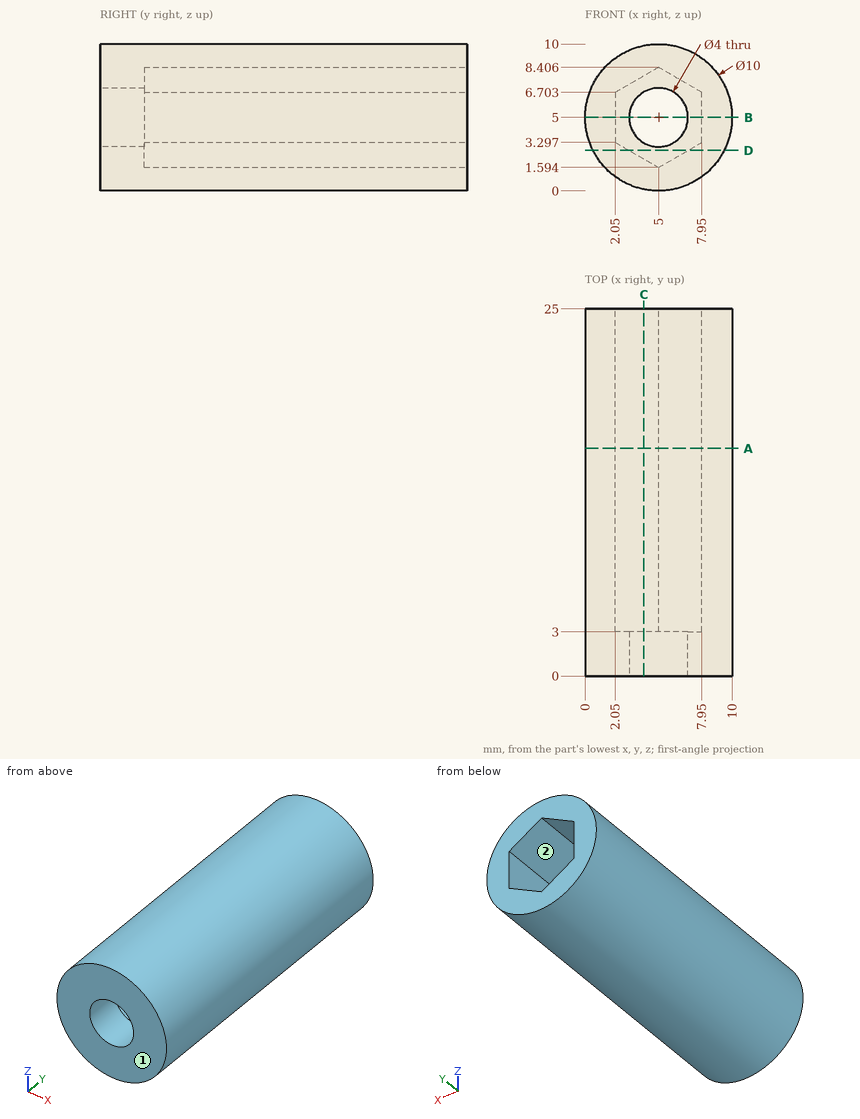
Geometry check sheet. Reference: drawing and pictorial views, mm from the part's lowest x, y, z. A direction names the side the tool comes from. Round coordinates to 2 decimals unless told otherwise and drop trailing zeros. Loops run counter-clockwise (first coordinate to the right, second up) from the corner with the lowest first, then second, coordinate; pieces in that order, holes last. Notation, with made-up numbers: (43.25, -25.75) -> (79.25, -25.75) arc R9 ccw to (79.25, -11.75) -> close; hole circle Ø1 at (11, -35.5). An arc over 180 degrees is marked (long way). Answer as a JSON object with one key per item and string values.
Q1. Section check A-A (y = 15.5). Record the boundary of the cut face in (x, z).
Data:
{"outline": "circle Ø10 at (5, 5); hole (2.05, 3.3) -> (5, 1.59) -> (7.95, 3.3) -> (7.95, 6.7) -> (5, 8.41) -> (2.05, 6.7) -> close"}
Q2. Go/stop test with flat-tipped pins: P1, Ø2, axis at x = 8.5, y = 13, coming from the +Z side; P2, Ø5, axis at x = 5, z = 5, coming from the +Y side; P3, Ø3, axis at y = 17, z = 8, coming from the +X side. Record where each tip stops, or that it passes through.
Data:
{"P1": "stops at z = 9.33", "P2": "stops at y = 3", "P3": "stops at x = 9.77"}
Q3. Access from +Z, -Z, +X, -X, +Y, -Y to the whole of each face (thin tool, end or side, straight path). Record for the marked faces 1 and 2.
Data:
{"face 1": "+Z, -Z, +X, -X, -Y", "face 2": "+Y"}
Q4. Section check B-B (z = 5). Record the boundary of the cut face in (x, y), then the cut area to 3 significant figures.
Data:
{"outline": "(0, 0) -> (3, 0) -> (3, 3) -> (2.05, 3) -> (2.05, 25) -> (0, 25) -> close; (7, 0) -> (10, 0) -> (10, 25) -> (7.95, 25) -> (7.95, 3) -> (7, 3) -> close", "area": "108 mm2"}
Q5. Section check D-D (z = 2.75). Record the boundary of the cut face in (x, y) (1 decimal).
Data:
{"outline": "(0.5, 0) -> (9.5, 0) -> (9.5, 25) -> (7, 25) -> (7, 3) -> (3, 3) -> (3, 25) -> (0.5, 25) -> close"}
Q6. Scan lines: line 1 (Z direction, x = 5, y = 2); line 2 (X direction, y = 8.75, z = 6.5); line 3 (Z direction, x = 3, y = 6.25). Record each from-to range of solid material in increasing order. Write a range as from..to.
Data:
{"line 1": "z = 0..3, 7..10", "line 2": "x = 0.23..2.05, 7.95..9.77", "line 3": "z = 0.42..2.75, 7.25..9.58"}
Q7. Section check C-C (x = 4). Record the boundary of the cut face in (y, z).
Data:
{"outline": "(0, 0.1) -> (25, 0.1) -> (25, 2.17) -> (3, 2.17) -> (3, 3.27) -> (0, 3.27) -> close; (0, 6.73) -> (3, 6.73) -> (3, 7.83) -> (25, 7.83) -> (25, 9.9) -> (0, 9.9) -> close"}
